Source: three-view drawing plus pictorial views. Frame: mm from the lowest corner of the part. A direction names the side the tool comes from. Coordinates: 2 decimals unless noted, no trailing zeros. Write each loop counter-clockwise with the first axis right and the second up, starting at its lowest first coordinate (ties: lowest second). Pieces come first, ordered by that corner, then holes. Notation, with made-up numbers: (84.5, 2) -> (91.5, 2) arc R23 cw to (91.5, 27) -> close; hole circle Ø11 at (-9.75, -30). An arc over 180 degrees is marked (long way). Write item = value, one per line.
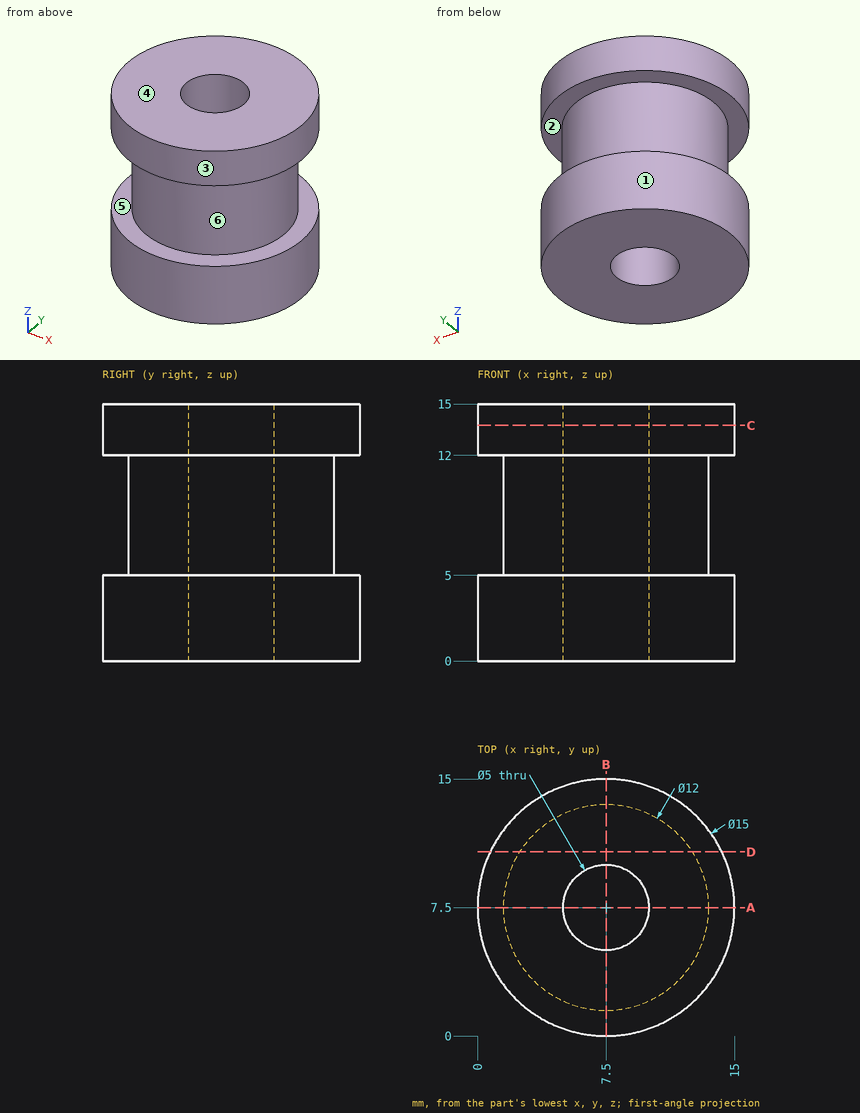
1) Cut plane C-C, the plane z = 13.75. Output: boundary loops of the cut face in (x, y), and give its area (3 significant figures).
Answer block:
outline = circle Ø15 at (7.5, 7.5); hole circle Ø5 at (7.5, 7.5)
area = 157 mm2
2) Reachability of the marked faces 1 and 2 from +Z, -Z, +X, -X, +Y, -Y: full face, straight path, thin tool, end or side. Return the list, or none.
Answer block:
face_1 = +Z, -Z
face_2 = none
3) Pull-direction query (Z, two-part tool) for the marked faces 3, 4, 5 and 6; classes: +Z half, -Z half, draft (parallel to the pull), parting line (faces both ways), or undercut.
Answer block:
face_3 = draft
face_4 = +Z half
face_5 = undercut
face_6 = undercut
4) First-contact query: pin 1 Ø4 at (y, z) = (2, 12.5) entering from -X; pin 2 Ø4 at (y, z) = (12, 11.5) entering from -X; pin 3 Ø3 at (x, z) = (2, 9) entering from -Y. Flat tips, straight axial feed; report the tip coordinate or a pass-through.
Answer block:
pin_1 = 0.87
pin_2 = 0.45
pin_3 = 3.03
5) Material intervals for probe 1 along Y at (x, z) = (7.5, 7.5); probe 2 along Z at (x, y) = (12.25, 13.25); probe 3 along Y at (x, z) = (9.75, 6.25), sorted ascending. Write a range as [from, to].
Answer block:
probe_1 = [1.5, 5], [10, 13.5]
probe_2 = [0, 5], [12, 15]
probe_3 = [1.94, 6.41], [8.59, 13.06]
6) Cut plane D-D, the plane y = 10.75. Output: boundary loops of the cut face in (x, z), and give its area (3 significant figures).
Answer block:
outline = (0.74, 0) -> (14.26, 0) -> (14.26, 5) -> (12.54, 5) -> (12.54, 12) -> (14.26, 12) -> (14.26, 15) -> (0.74, 15) -> (0.74, 12) -> (2.46, 12) -> (2.46, 5) -> (0.74, 5) -> close
area = 179 mm2
7) Cut plane A-A, the plane y = 7.5. Output: boundary loops of the cut face in (x, z), and give its area (3 significant figures).
Answer block:
outline = (0, 0) -> (5, 0) -> (5, 15) -> (0, 15) -> (0, 12) -> (1.5, 12) -> (1.5, 5) -> (0, 5) -> close; (10, 0) -> (15, 0) -> (15, 5) -> (13.5, 5) -> (13.5, 12) -> (15, 12) -> (15, 15) -> (10, 15) -> close
area = 129 mm2
